The model under review builds one solid part; all positions refer to its coordinate system, in mm. A direction names the side the tool comes from. Round coordinates to 2 decimals unless told otherwise and drop trailing zeros. Write each loop counter-clockwise with the first axis right and the second up, starting at its lowest first coordinate (ties: lowest second). Pieces come first, ordered by that corner, then holes. Notation, with made-up numbers: (78, 25.25) -> (100, 25.25) arc R12 cw to (100, 34.25) -> close; hole circle Ø3 at (39, 34). An arc over 180 degrees is marked (long way). Return JSON: item names as keys, results as strings. Group by question number.
1. Take a section at A-A, the plane z = 1.55. Write out the cut boundary in (x, y).
2. Clearance check with flat-ended pins moving along their axes: P1, Ø1.5, axis at x = 1.5, z = 3, coming from the +Y side; P2, Ø2.5, axis at x = 6.5, z = 2, coming from the +Y side; P3, Ø1.5, axis at y = 43, z = 3.5, coming from the +X side. State where each tip first meets the part, or that it passes through.
3. Take a section at C-C, the plane y = 29. Write out the cut boundary in (x, z), then the cut area to 3 significant figures.
4. Take a section at B-B, the plane x = 6. Write out the cut boundary in (y, z), then the cut area to 3 significant figures.
5. For line 1 along Y through (x, z) = (0, 2.35); line 2 along Y through (x, z) = (8.25, 2.4); line 3 along X through (y, z) = (24.5, 1.25), list the stretches that pass through material, from the lowest coordinate up. Write a range as from..to.
6. Tool access review of faces 1 (the flat face through (2, 40, 2)), 2 (the flat face through (-2, 41, 2)): name each direction out of +Z, -Z, +X, -X, +Y, -Y from which nothing blocks a thin tool from reaching the whole face with its end or side.
7. Mouldability with a two-part tool opening along Y and no side actions: class faces 3 (the cylindrical face through (7.46, -0.61, 2.46)), 4 (the cylindrical face through (10.243, -0.167, 2.465)), 5 (the cylindrical face through (0, -1, 2)), 6 (the flat face through (0, 40, 5)) as pulls with the +Y half, pulls with the -Y half, needs draft (parallel to the pull), parting line crosses it, or undercut.
from build123d import *

# Parameters (mm, degrees)
SKETCH_1_R      = 1
EXTRUDE_1_DEPTH = 5


with BuildPart() as part:
    # 草图1 → 凸台-拉伸1 (new body)
    with BuildSketch(Plane.XY):
        with BuildLine():
            Line((-2, 80), (-2, 0))
            ThreePointArc((-2, 0), (-1.414213562, -1.414213562), (0, -2))
            Line((0, -2), (8.25, -2))
            ThreePointArc((8.25, -2), (10.246076458, -0.125214915), (8.499938543, 1.984321225))
            Line((8.499938543, 1.984321225), (1.999938543, 1.984321225))
            Line((1.999938543, 1.984321225), (1.999938543, 79.984321225))
            ThreePointArc((1.999938543, 79.984321225), (0.007839448, 81.999984636), (-2, 80))
        make_face()
        Circle(SKETCH_1_R, mode=Mode.SUBTRACT)
        with Locations((8.25, 0)):
            Circle(SKETCH_1_R, mode=Mode.SUBTRACT)
    extrude(amount=EXTRUDE_1_DEPTH)


solid = part.part
Output:
{
 "1": {"outline": "(-2, 0) arc R2 ccw to (0, -2) -> (8.25, -2) arc R2 ccw to (8.5, 1.98) -> (2, 1.98) -> (2, 79.98) arc R2 ccw (long way) to (-2, 80) -> close; hole circle Ø2 at (0, 0); hole circle Ø2 at (8.25, 0)"},
 "2": {"P1": "stops at y = 81.85", "P2": "stops at y = 1.98", "P3": "stops at x = 2"},
 "3": {"outline": "(-2, 0) -> (2, 0) -> (2, 5) -> (-2, 5) -> close", "area": "20.0 mm^2"},
 "4": {"outline": "(-2, 0) -> (1.98, 0) -> (1.98, 5) -> (-2, 5) -> close", "area": "19.9 mm^2"},
 "5": {"line 1": "y = -2..-1, 1..82", "line 2": "y = -2..-1, 1..1.98", "line 3": "x = -2..2"},
 "6": {"face 1": "+Z, -Z, +X, +Y", "face 2": "+Z, -Z, -X, +Y, -Y"},
 "7": {"face 3": "undercut", "face 4": "parting line crosses it", "face 5": "undercut", "face 6": "needs draft"}
}
